Could you check a few things on this model? Use its own coordinates, in mm. A direction names the side the tool comes from. Coordinates: 2 decimals unless noted, no trailing zeros. Order: outer loops, then holes, each group sorted by start corner. A loop starts at its lowest first (then second) coordinate and runs counter-clockwise, first axis right, second up.
```python
from build123d import *

# Parameters (mm, degrees)
F0_R     = 14
F1_DEPTH = 40
F3_D     = 18
F3_DEPTH = 7.3
F3_TIP   = 5.4077455712
F4_D     = 11
F4_DEPTH = 15
F4_TIP   = 3.3047334047


with BuildPart() as f1:
    # F0 (on Front) → F1 (new body)
    with BuildSketch(Plane.XZ):
        with BuildLine():
            Line((-55, 15), (-55, 0))
            Line((-55, 0), (55, 0))
            Line((55, 0), (55, 15))
            Line((55, 15), (25, 15))
            Line((25, 15), (25, 49.7154739381))
            Line((25, 49.7154739381), (24.9280575663, 49.8561188579))
            ThreePointArc((24.9280575663, 49.8561188579), (0, 65.1049641661), (-24.9280575663, 49.8561188579))
            Line((-24.9280575663, 49.8561188579), (-25, 49.7154739381))
            Line((-25, 49.7154739381), (-25, 15))
            Line((-25, 15), (-55, 15))
        make_face()
        with Locations((0, 40)):
            Circle(F0_R, mode=Mode.SUBTRACT)
    extrude(amount=F1_DEPTH)

    # F3
    with Locations(Plane.XY.offset(15)):
        with Locations((-40, -20), (40, -20)):
            Hole(F3_D / 2, depth=F3_DEPTH)
            with Locations((0, 0, -(F3_DEPTH + F3_TIP / 2))):  # 118° drill point
                Cone(0, F3_D / 2, F3_TIP, mode=Mode.SUBTRACT)

    # F4
    with Locations(Plane.XY.offset(15)):
        with Locations((-40, -20), (40, -20)):
            Hole(F4_D / 2, depth=F4_DEPTH)
            with Locations((0, 0, -(F4_DEPTH + F4_TIP / 2))):  # 118° drill point
                Cone(0, F4_D / 2, F4_TIP, mode=Mode.SUBTRACT)


solid = f1.part
```
Item 1: For pin 1 Ø5 at (y, z) = (-28.5, 28) entering from +X; pin 2 Ø6.5 at (x, y) = (40, -20) entering from +Z; pin 3 Ø8 at (x, y) = (35, -22) entering from +Z; pin 4 Ø12.5 at (x, y) = (-40, -20) entering from +Z, each with a flat end and sliding along its axis, tell me the tip position at first contact or that it passes through.
Item 2: Suppose I cut it at B-B (y = -20). List the corners of the cut face in (x, z) for me, and give its area (3 significant figures).
Item 3: Thinking about a two-plate mould opening in X: for faces 1 (the face through (-3.03, -19.72, 26.33)), 2 (the face through (-39.8, -10.8, 15)), 3 (the face through (0.43, -19.72, 65.1)), which applies, +X half, -X half, draft (parallel to the pull), parting line (faces both ways), or undercut?
Item 4: Which directions (+Z, -Z, +X, -X, +Y, -Y) give clear straight access to the entire face, cutting with the end or side of a thin tool? Please do faces 4 (the face through (49, -20, 11)), 5 (the face through (-55, -20, 8)), 6 (the face through (-25, -20, 33)), 7 (the face through (25, -20, 32)).
Item 5: Suppose I cut it at A-A (x = -40). List the corners of the cut face in (y, z) for me, and give its area (3 significant figures).
Item 6: Suppose I cut it at C-C (z = 12). List the corners of the cut face in (x, y) for me, and give its area (3 significant figures).
Item 7: Suppose I cut it at D-D (y = -36). List the corners of the cut face in (x, z) for me, and give its area (3 significant figures).
Item 8: I need wall thicknesses on line 1 (X direction, y = -20, z = 10.25); line 2 (X direction, y = -20, z = 3); line 3 (Z direction, x = 0, y = -30.5). Which ranges of each line are inside material? Lowest first, please.
Geometry results:
1. pin 1: stops at x = 25
1. pin 2: passes through
1. pin 3: stops at z = 15
1. pin 4: stops at z = 6.05
2. outline: (-55, 0) - (-45.5, 0) - (-45.5, 5.6) - (-49, 7.7) - (-49, 15) - (-55, 15) - close; (-34.5, 0) - (34.5, 0) - (34.5, 5.6) - (31, 7.7) - (31, 15) - (25, 15) - (25, 49.72) - (24.93, 49.86) arc R28 ccw to (-24.93, 49.86) - (-25, 49.72) - (-25, 15) - (-31, 15) - (-31, 7.7) - (-34.5, 5.6) - close; (45.5, 0) - (55, 0) - (55, 15) - (49, 15) - (49, 7.7) - (45.5, 5.6) - close; hole circle Ø28 at (0, 40)
2. area: 2,870 mm2
3. face 1: undercut
3. face 2: draft
3. face 3: parting line
4. face 4: +Z
4. face 5: +Z, -Z, -X, +Y, -Y
4. face 6: +Z, -X, +Y, -Y
4. face 7: +Z, +X, +Y, -Y
5. outline: (-40, 0) - (-25.5, 0) - (-25.5, 5.6) - (-29, 7.7) - (-29, 15) - (-40, 15) - close; (-14.5, 0) - (0, 0) - (0, 15) - (-11, 15) - (-11, 7.7) - (-14.5, 5.6) - close
5. area: 377 mm2
6. outline: (-55, -40) - (55, -40) - (55, 0) - (-55, 0) - close; hole circle Ø18 at (-40, -20); hole circle Ø18 at (40, -20)
6. area: 3,890 mm2
7. outline: (-55, 0) - (55, 0) - (55, 15) - (25, 15) - (25, 49.72) - (24.93, 49.86) arc R28 ccw to (-24.93, 49.86) - (-25, 49.72) - (-25, 15) - (-55, 15) - close; hole circle Ø28 at (0, 40)
7. area: 3,320 mm2
8. line 1: x = -55 to -49, -31 to 31, 49 to 55
8. line 2: x = -55 to -45.5, -34.5 to 34.5, 45.5 to 55
8. line 3: z = 0 to 26, 54 to 65.1
